Autodesk Inventor part; units mm, degrees
ref_plane "YZ Plane" through (0, 0, 0) normal (1, 0, 0) x (0, 1, 0)
ref_plane "XZ Plane" through (0, 0, 0) normal (0, 1, 0) x (-1, 0, 0)
ref_plane "XY Plane" through (0, 0, 0) normal (0, 0, 1) x (1, 0, 0)
sketch "Sketch1" plane through (0, 0, 0) normal (0, 1, 0) x (-1, 0, 0)
  circle A0 centre (0, 0) radius 1.143
  dimension "d24" = 2.286
extrude "Extrusion1" add sketch "Sketch1" along normal blind 12.5
sketch "Sketch2" plane through (0, 12.5, 0) normal (0, 1, 0) x (1, 0, 0)
  circle A0 centre (0, 0) radius 1.5
  circle A1 centre (0, 0) radius 2.54
  dimension "d3" = 5.08
extrude "Extrusion2" add sketch "Sketch2" along normal blind 3 contours A0 | A1
fillet "Fillet1" radius 0.508 2 edges at (-2.54, 15.5, 0) (-2.54, 12.5, 0)
sketch "Sketch3" plane through (0, 15.5, 0) normal (0, 1, 0) x (1, 0, 0)
  line L0 (0, 0) -> (1.5, 0) construction
  line L1 (-1.299, -0.75) -> (-1.299, 0.75)
  line L2 (-1.299, 0.75) -> (0.0002, 1.5)
  line L3 (1.299, 0.75) -> (0.0002, 1.5)
  line L4 (1.299, 0.75) -> (1.299, -0.75)
  line L5 (0, -1.5) -> (1.299, -0.75)
  line L6 (-1.299, -0.75) -> (0, -1.5)
extrude "Extrusion4" cut sketch "Sketch3" against normal blind 1
sketch "Sketch4" plane through (0, 0, 0) normal (0, 0, 1) x (1, 0, 0)
  point P0 (0, 0)
sketch "Sketch5" plane through (0, 0, 0) normal (0, -1, 0) x (1, 0, 0)
  circle A0 centre (0, 0) radius 3.3551
extrude "Extrusion5" cut sketch "Sketch5" against normal blind 5.715
thread "Thread3"
properties part number "screw"
For this review, take the finished solid that the model builds, in its own axes (mm). A direction names the side the tool comes from. Round coordinates to 2 decimals unless told otherwise and drop trailing zeros. Write each loop counter-clockwise with the first axis right and the second up, starting at its lowest first coordinate (ties: lowest second). Pieces come first, ordered by that corner, then holes. Notation, with made-up numbers: (82, 8.25) -> (120, 8.25) arc R15 cw to (120, 22.25) -> close; hole circle Ø6 at (10.25, 70.25). An arc over 180 degrees is marked (long way). Use CSV: the item, a comma, the result in double quotes.
(1) For faces 4 (the face through (0.66, 15.01, -1.12)), 5 (the face through (1, 12.5, 1)), list the 3-axis set-ups (+Z, -Z, +X, -X, +Y, -Y) from which the entire face can be reached by the end or side of a thin tool; tool diameter is ignored.
Computed values:
face 4,"+Y"
face 5,"-Y"
(2) Consider section B-B, the plane z = 0. Give the boundary of the cut face in (x, y) (3 decimals), plus the area to 3 significant figures.
Computed values:
outline,"(-2.54, 13.008) arc R0.508 ccw to (-2.032, 12.5) -> (-1.143, 12.5) -> (-1.143, 5.715) -> (1.143, 5.715) -> (1.143, 12.5) -> (2.032, 12.5) arc R0.508 ccw to (2.54, 13.008) -> (2.54, 14.992) arc R0.508 ccw to (2.032, 15.5) -> (1.299, 15.5) -> (1.299, 14.5) -> (-1.299, 14.5) -> (-1.299, 15.5) -> (-2.032, 15.5) arc R0.508 ccw to (-2.54, 14.992) -> close"
area,"27.9 mm²"
(3) To check wall thickness, follow L1, parallel to Y at x = -0.05, z = 0.45 (3 decimals); L2, parallel to Y at x = 1.7, z = -0.35; L3, parallel to X at y = 14.75, z = 0.5. State the ranges of each line that lie inside material, in increasing order. Write a range as [from, to].
Computed values:
L1,"[5.715, 14.5]"
L2,"[12.5, 15.5]"
L3,"[-2.49, -1.3], [1.3, 2.49]"
(4) Consider section A-A, the plane y = 14.75. Give the boundary of the cut face in (x, z).
Computed values:
outline,"circle Ø5.08 at (0, 0); hole (-1.3, -0.75) -> (0, -1.5) -> (1.3, -0.75) -> (1.3, 0.75) -> (0, 1.5) -> (-1.3, 0.75) -> close"
(5) Clearance check with flat-ended pins moving along their axes: P1, Ø3, axis at y = 9, z = 1.5, coming from the -X side; P2, Ø1, axis at x = -0.5, y = 10.5, coming from the -Z side. State where each tip first meets the part, or that it passes through.
Computed values:
P1,"x = -1.14"
P2,"z = -1.14"
(6) Draft analysis for pull direction Z (two halves, no side actions). For faces 1 (the face through (-0.33, 13.99, 2.52)), 2 (the face through (0, 14.5, 0)), 3 (the face through (0, 5.715, 0)), state which applies: +Z half, -Z half, draft (parallel to the pull), parting line (faces both ways), or undercut.
Computed values:
face 1,"parting line"
face 2,"undercut"
face 3,"draft"
(7) Consider section C-C, the plane y = 8.75. Give the boundary of the cut face in (x, z), plus the area to 3 significant figures.
Computed values:
outline,"circle Ø2.29 at (0, 0)"
area,"4.10 mm²"
